from build123d import *

# Parameters (mm, degrees)
SKETCH1_W           = 10
SKETCH1_H           = 10
SKETCH1_R           = 7.5
SKETCH1_R_2         = 2.25
BOSS_EXTRUDE1_DEPTH = 5
SKETCH2_W           = 10
SKETCH2_H           = 10
BOSS_EXTRUDE2_DEPTH = 26
SKETCH4_R           = 2
BOSS_EXTRUDE3_DEPTH = 3
FILLET1_R           = 1
SKETCH5_R           = 3.25
CUT_EXTRUDE1_DEPTH  = 2


with BuildPart() as part:
    # Sketch1 → Boss-Extrude1 (new body)
    # profile 1 of 5: a face of its own
    with BuildSketch(Plane.XY):
        with Locations((-14.5, 20.85)):
            Rectangle(SKETCH1_W, SKETCH1_H)
    # profile 2 of 5: a face of its own
    with BuildSketch(Plane.XY):
        with Locations((14.5, 20.85)):
            Rectangle(SKETCH1_W, SKETCH1_H)
    # profile 3 of 5: a face of its own
    with BuildSketch(Plane.XY):
        with BuildLine():
            Line((-20.5, -1.457145002), (-20.5, -14.85))
            ThreePointArc((-20.5, -14.85), (-20.207106781, -15.557106781), (-19.5, -15.85))
            Line((-19.5, -15.85), (19.5, -15.85))
            ThreePointArc((19.5, -15.85), (20.207106781, -15.557106781), (20.5, -14.85))
            Line((20.5, -14.85), (20.5, 14.85))
            ThreePointArc((20.5, 14.85), (20.207106781, 15.557106781), (19.5, 15.85))
            Line((19.5, 15.85), (-19.5, 15.85))
            ThreePointArc((-19.5, 15.85), (-20.207106781, 15.557106781), (-20.5, 14.85))
            Line((-20.5, 14.85), (-20.5, -1.457145002))
        make_face()
        with Locations((6.9, 0)):
            Circle(SKETCH1_R, mode=Mode.SUBTRACT)
        with Locations((15.5, 8.3)):
            Circle(SKETCH1_R_2, mode=Mode.SUBTRACT)
        with Locations((15.5, -8.3)):
            Circle(SKETCH1_R_2, mode=Mode.SUBTRACT)
        with Locations((-15.5, -8.3)):
            Circle(SKETCH1_R_2, mode=Mode.SUBTRACT)
        with Locations((-15.5, 8.3)):
            Circle(SKETCH1_R_2, mode=Mode.SUBTRACT)
    # profile 4 of 5: a face of its own
    with BuildSketch(Plane.XY):
        with Locations((14.5, -20.85)):
            Rectangle(SKETCH1_W, SKETCH1_H)
    # profile 5 of 5: a face of its own
    with BuildSketch(Plane.XY):
        with Locations((-14.5, -20.85)):
            Rectangle(SKETCH1_W, SKETCH1_H)
    extrude(amount=BOSS_EXTRUDE1_DEPTH)

    # Sketch2 → Boss-Extrude2 (add)
    with BuildSketch(Plane(origin=(0, 0, 0), x_dir=(-1, 0, 0), z_dir=(0, 0, -1))):
        with Locations((14.5, -20.85)):
            Rectangle(SKETCH2_W, SKETCH2_H)
        with Locations((-14.5, -20.85)):
            Rectangle(SKETCH2_W, SKETCH2_H)
        with Locations((14.5, 20.85)):
            Rectangle(SKETCH2_W, SKETCH2_H)
        with Locations((-14.5, 20.85)):
            Rectangle(SKETCH2_W, SKETCH2_H)
    extrude(amount=BOSS_EXTRUDE2_DEPTH)

    # Sketch4 → Boss-Extrude3 (add)
    # profile 1 of 4: a face of its own
    with BuildSketch(Plane(origin=(0, 0, -26), x_dir=(-1, 0, 0), z_dir=(0, 0, -1))):
        with BuildLine():
            Line((9.5, -25.85), (9.5, -35.647958971))
            ThreePointArc((9.5, -35.647958971), (14.5, -36.85), (19.5, -35.647958971))
            Line((19.5, -35.647958971), (19.5, -25.85))
            Line((19.5, -25.85), (9.5, -25.85))
        make_face()
        with Locations((14.5, -31.35)):
            Circle(SKETCH4_R, mode=Mode.SUBTRACT)
    # profile 2 of 4: a face of its own
    with BuildSketch(Plane(origin=(0, 0, -26), x_dir=(-1, 0, 0), z_dir=(0, 0, -1))):
        with BuildLine():
            Line((-19.5, -25.85), (-19.5, -35.647958971))
            ThreePointArc((-19.5, -35.647958971), (-14.5, -36.85), (-9.5, -35.647958971))
            Line((-9.5, -35.647958971), (-9.5, -25.85))
            Line((-9.5, -25.85), (-19.5, -25.85))
        make_face()
        with Locations(Location((-14.5, -31.35, 0), (0, 0, 180))):
            Circle(SKETCH4_R, mode=Mode.SUBTRACT)
    # profile 3 of 4: a face of its own
    with BuildSketch(Plane(origin=(0, 0, -26), x_dir=(-1, 0, 0), z_dir=(0, 0, -1))):
        with BuildLine():
            Line((19.5, 25.85), (19.5, 35.647958971))
            ThreePointArc((19.5, 35.647958971), (14.5, 36.85), (9.5, 35.647958971))
            Line((9.5, 35.647958971), (9.5, 25.85))
            Line((9.5, 25.85), (19.5, 25.85))
        make_face()
        with Locations(Location((14.5, 31.35, 0), (0, 0, 180))):
            Circle(SKETCH4_R, mode=Mode.SUBTRACT)
    # profile 4 of 4: a face of its own
    with BuildSketch(Plane(origin=(0, 0, -26), x_dir=(-1, 0, 0), z_dir=(0, 0, -1))):
        with BuildLine():
            Line((-9.5, 25.85), (-9.5, 35.647958971))
            ThreePointArc((-9.5, 35.647958971), (-14.5, 36.85), (-19.5, 35.647958971))
            Line((-19.5, 35.647958971), (-19.5, 25.85))
            Line((-19.5, 25.85), (-9.5, 25.85))
        make_face()
        with Locations((-14.5, 31.35)):
            Circle(SKETCH4_R, mode=Mode.SUBTRACT)
    extrude(amount=-BOSS_EXTRUDE3_DEPTH)

    # Fillet1
    fillet1_edges = [part.edges().sort_by_distance(p)[0] for p in [
        (9.5, 25.85, -9),
        (19.5, 25.85, -9),
        (19.5, -25.85, -9),
        (9.5, -25.85, -9),
        (-9.5, -25.85, -9),
        (-19.5, -25.85, -9),
        (-19.5, 25.85, -9),
        (-9.5, 25.85, -9),
    ]]
    fillet(fillet1_edges, radius=FILLET1_R)

    # Sketch5 → Cut-Extrude1 (cut)
    with BuildSketch(Plane.XY.offset(5)):
        with Locations((-15.5, -8.3)):
            Circle(SKETCH5_R)
        with Locations((-15.5, 8.3)):
            Circle(SKETCH5_R)
        with Locations((15.5, -8.3)):
            Circle(SKETCH5_R)
        with Locations(Location((15.5, 8.3, 0), (0, 0, 180))):
            Circle(SKETCH5_R)
    extrude(amount=-CUT_EXTRUDE1_DEPTH, mode=Mode.SUBTRACT)


solid = part.part
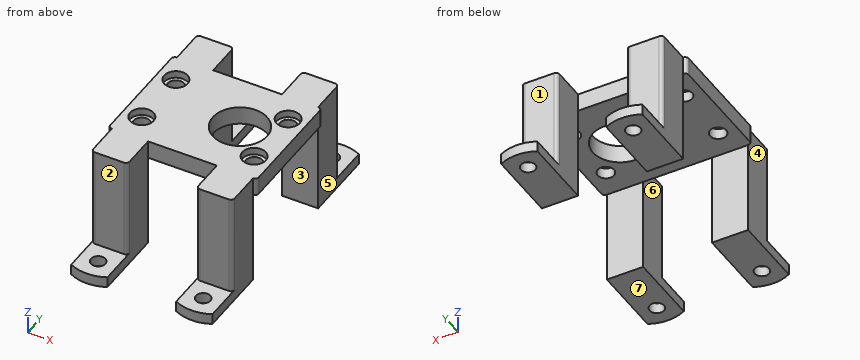
Source: CAD feature listing. Evaluate the final solid. Frame: model axes, mm. Face numbers are marked on the shaded views. A direction names the side the tool comes from. Round coordinates to 2 decimals unless told otherwise and drop trailing zeros. Loops run counter-clockwise (first coordinate to the right, second up) from the corner with the lowest first, then second, coordinate; pieces in that order, holes last. Notation, with made-up numbers: (54.5, 18.5) - (84.5, 18.5) arc R25 cw to (84.5, 32.5) - close; hole circle Ø2 at (64, 68.25). An arc over 180 degrees is marked (long way). Write item = value, one per line. Start each with the question number.
Item 1: Section query B-B on x = 6.9. Output: boundary loops of the cut face in (y, z), plus the area to 3 significant figures.
Item 2: Section query A-A on y = -8.3. Output: boundary loops of the cut face in (x, z), plus the area to 3 significant figures.
Item 3: Material intervals for line 1 (X direction, y = -8.3, z = 2.05); line 2 (X direction, y = 23, z = -12.5); line 3 (Y direction, x = -13.5, z = -21), sorted ascending.
Item 4: Mould query, pull axis X, two halves, no side actions, for the marked faces 4, 5, 6 and 7. Classes: released by +X, released by -X, zero draft, split by the parting line, or undercut.
Item 5: Section query D-D on x = -15.5. Count the separate pieces of the cut face and the enclosed holes in it, plus the area to 3 significant figures.
Item 6: Reachability of the marked faces 1, 2 and 3 from +Z, -Z, +X, -X, +Y, -Y: full face, straight path, thin tool, end or side. Return the list, or none.
Item 7: Section query C-C on y = 31.35. Output: boundary loops of the cut face in (x, z).
Item 8: First-contact query: pin 1 Ø10 at (y, z) = (-25.5, -15) entering from +X; pin 2 Ø6.5 at (x, z) = (-16, -11.5) entering from -Y; pin 3 Ø3 at (x, y) = (-13, 33) entering from +Z. Flat tips, straight axial feed; report the tip coordinate or a pass-through.
Results list:
q1.outline = (-15.85, 0) - (-7.5, 0) - (-7.5, 5) - (-15.85, 5) - close; (7.5, 0) - (15.85, 0) - (15.85, 5) - (7.5, 5) - close
q1.area = 83.5 mm²
q2.outline = (-20.5, 0) - (-17.75, 0) - (-17.75, 3) - (-18.75, 3) - (-18.75, 5) - (-20.5, 5) - close; (-13.25, 0) - (13.25, 0) - (13.25, 3) - (12.25, 3) - (12.25, 5) - (-12.25, 5) - (-12.25, 3) - (-13.25, 3) - close; (17.75, 0) - (20.5, 0) - (20.5, 5) - (18.75, 5) - (18.75, 3) - (17.75, 3) - close
q2.area = 152 mm²
q3.line_1 = -20.5 to -17.75, -13.25 to 13.25, 17.75 to 20.5
q3.line_2 = -19.5 to -9.5, 9.5 to 19.5
q3.line_3 = -25.85 to -15.85, 15.85 to 25.85
q4.face_4 = released by -X
q4.face_5 = released by +X
q4.face_6 = undercut
q4.face_7 = zero draft
q5.separate_pieces = 5
q5.enclosed_holes = 0
q5.area = 770 mm²
q6.face_1 = +Z, +X, -X, +Y
q6.face_2 = +Z, +X, -X, -Y
q6.face_3 = -Z, +X, -X
q7.outline = (-19.5, -26) - (-16.5, -26) - (-16.5, -23) - (-19.5, -23) - close; (-12.5, -26) - (-9.5, -26) - (-9.5, -23) - (-12.5, -23) - close; (9.5, -26) - (12.5, -26) - (12.5, -23) - (9.5, -23) - close; (16.5, -26) - (19.5, -26) - (19.5, -23) - (16.5, -23) - close
q8.pin_1 = 19.5
q8.pin_2 = -25.85
q8.pin_3 = -23
